The listing builds one solid part. Answer for the finished solid, in the listing's coordinates (mm). Round coordinates to 2 decimals unless told otherwise and drop trailing zeros. Write each loop counter-clockwise with the first axis right and the second up, starting at its lowest first coordinate (ties: lowest second). Pieces come first, ordered by that corner, then holes. Notation, with made-up numbers: (12.5, 37.5) - (49.5, 37.5) arc R17 cw to (49.5, 43.5) - close; hole circle Ø10 at (27.5, 58). An arc over 180 degrees is marked (long way). Return JSON: item names as keys, results as strings. Group by question number.
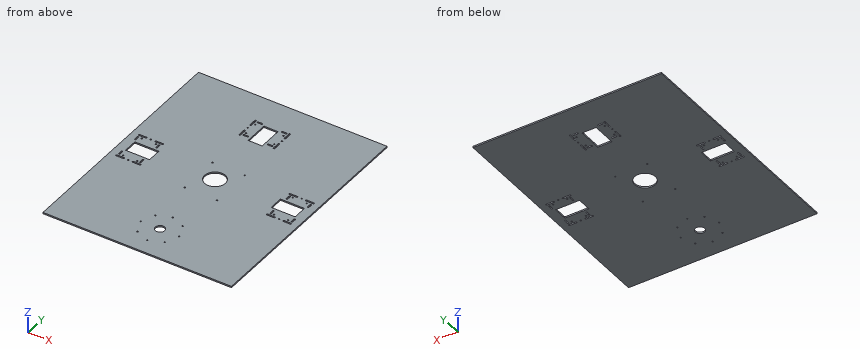
from build123d import *

# Parameters (mm, degrees)
SKETCH_1_W          = 400
SKETCH_1_H          = 500
SKETCH_1_R          = 1.5
SKETCH_1_R_2        = 22
SKETCH_1_R_3        = 10
SKETCH_1_W_2        = 30
SKETCH_1_H_2        = 51
SKETCH_1_W_3        = 51
SKETCH_1_H_3        = 30
EXTRUDE_1_DEPTH     = 3
SKETCH_2_R          = 1.5
CUT_EXTRUDE_1_DEPTH = 321.170267202


with BuildPart() as part:
    # 草图1 → 凸台-拉伸1 (new body)
    with BuildSketch(Plane.XY):
        Rectangle(SKETCH_1_W, SKETCH_1_H)
        with Locations((-36.4, 160)):
            Circle(SKETCH_1_R, mode=Mode.SUBTRACT)
        with Locations((-30, 145)):
            Circle(SKETCH_1_R, mode=Mode.SUBTRACT)
        with Locations((-30, 175)):
            Circle(SKETCH_1_R, mode=Mode.SUBTRACT)
        with Locations((36.4, 160)):
            Circle(SKETCH_1_R, mode=Mode.SUBTRACT)
        with Locations((30, 175)):
            Circle(SKETCH_1_R, mode=Mode.SUBTRACT)
        with Locations((30, 145)):
            Circle(SKETCH_1_R, mode=Mode.SUBTRACT)
        with Locations((160, -36.4)):
            Circle(SKETCH_1_R, mode=Mode.SUBTRACT)
        with Locations((145, -30)):
            Circle(SKETCH_1_R, mode=Mode.SUBTRACT)
        with Locations((175, -30)):
            Circle(SKETCH_1_R, mode=Mode.SUBTRACT)
        with Locations((160, 36.4)):
            Circle(SKETCH_1_R, mode=Mode.SUBTRACT)
        with Locations((175, 30)):
            Circle(SKETCH_1_R, mode=Mode.SUBTRACT)
        with Locations((145, 30)):
            Circle(SKETCH_1_R, mode=Mode.SUBTRACT)
        with Locations((-160, 36.4)):
            Circle(SKETCH_1_R, mode=Mode.SUBTRACT)
        with Locations((-145, 30)):
            Circle(SKETCH_1_R, mode=Mode.SUBTRACT)
        with Locations((-175, 30)):
            Circle(SKETCH_1_R, mode=Mode.SUBTRACT)
        with Locations((-160, -36.4)):
            Circle(SKETCH_1_R, mode=Mode.SUBTRACT)
        with Locations((-175, -30)):
            Circle(SKETCH_1_R, mode=Mode.SUBTRACT)
        with Locations((-145, -30)):
            Circle(SKETCH_1_R, mode=Mode.SUBTRACT)
        Circle(SKETCH_1_R_2, mode=Mode.SUBTRACT)
        with Locations((0, -176.690492226)):
            Circle(SKETCH_1_R_3, mode=Mode.SUBTRACT)
        with Locations((0, -135.985304682)):
            Circle(SKETCH_1_R, mode=Mode.SUBTRACT)
        with Locations((28.782914142, -147.907578084)):
            Circle(SKETCH_1_R, mode=Mode.SUBTRACT)
        with Locations((40.705187545, -176.690492226)):
            Circle(SKETCH_1_R, mode=Mode.SUBTRACT)
        with Locations((28.782914142, -205.473406369)):
            Circle(SKETCH_1_R, mode=Mode.SUBTRACT)
        with Locations((0, -217.395679771)):
            Circle(SKETCH_1_R, mode=Mode.SUBTRACT)
        with Locations((-28.782914142, -205.473406369)):
            Circle(SKETCH_1_R, mode=Mode.SUBTRACT)
        with Locations((-40.705187545, -176.690492226)):
            Circle(SKETCH_1_R, mode=Mode.SUBTRACT)
        with Locations((-28.782914142, -147.907578084)):
            Circle(SKETCH_1_R, mode=Mode.SUBTRACT)
        with BuildLine():
            Line((-34.8, 185), (-34.8, 170))
            ThreePointArc((-34.8, 170), (-36.4, 168.4), (-38, 170))
            Line((-38, 170), (-38, 185))
            ThreePointArc((-38, 185), (-36.4, 186.6), (-34.8, 185))
        make_face(mode=Mode.SUBTRACT)
        with BuildLine():
            Line((-38, 135), (-38, 150))
            ThreePointArc((-38, 150), (-36.4, 151.6), (-34.8, 150))
            Line((-34.8, 150), (-34.8, 135))
            ThreePointArc((-34.8, 135), (-36.4, 133.4), (-38, 135))
        make_face(mode=Mode.SUBTRACT)
        with BuildLine():
            Line((-22, 181.8), (-30, 181.8))
            ThreePointArc((-30, 181.8), (-31.6, 183.4), (-30, 185))
            Line((-30, 185), (-22, 185))
            ThreePointArc((-22, 185), (-20.4, 183.4), (-22, 181.8))
        make_face(mode=Mode.SUBTRACT)
        with BuildLine():
            Line((-30, 140), (-22, 140))
            ThreePointArc((-22, 140), (-20.4, 138.4), (-22, 136.8))
            Line((-22, 136.8), (-30, 136.8))
            ThreePointArc((-30, 136.8), (-31.6, 138.4), (-30, 140))
        make_face(mode=Mode.SUBTRACT)
        with BuildLine():
            Line((30, 140), (22, 140))
            ThreePointArc((22, 140), (20.4, 138.4), (22, 136.8))
            Line((22, 136.8), (30, 136.8))
            ThreePointArc((30, 136.8), (31.6, 138.4), (30, 140))
        make_face(mode=Mode.SUBTRACT)
        with BuildLine():
            Line((38, 135), (38, 150))
            ThreePointArc((38, 150), (36.4, 151.6), (34.8, 150))
            Line((34.8, 150), (34.8, 135))
            ThreePointArc((34.8, 135), (36.4, 133.4), (38, 135))
        make_face(mode=Mode.SUBTRACT)
        with BuildLine():
            Line((34.8, 185), (34.8, 170))
            ThreePointArc((34.8, 170), (36.4, 168.4), (38, 170))
            Line((38, 170), (38, 185))
            ThreePointArc((38, 185), (36.4, 186.6), (34.8, 185))
        make_face(mode=Mode.SUBTRACT)
        with BuildLine():
            Line((22, 181.8), (30, 181.8))
            ThreePointArc((30, 181.8), (31.6, 183.4), (30, 185))
            Line((30, 185), (22, 185))
            ThreePointArc((22, 185), (20.4, 183.4), (22, 181.8))
        make_face(mode=Mode.SUBTRACT)
        with Locations((0, 154.5)):
            Rectangle(SKETCH_1_W_2, SKETCH_1_H_2, mode=Mode.SUBTRACT)
        with Locations((154.5, 0)):
            Rectangle(SKETCH_1_W_3, SKETCH_1_H_3, mode=Mode.SUBTRACT)
        with BuildLine():
            Line((185, 34.8), (170, 34.8))
            ThreePointArc((170, 34.8), (168.4, 36.4), (170, 38))
            Line((170, 38), (185, 38))
            ThreePointArc((185, 38), (186.6, 36.4), (185, 34.8))
        make_face(mode=Mode.SUBTRACT)
        with BuildLine():
            Line((135, 38), (150, 38))
            ThreePointArc((150, 38), (151.6, 36.4), (150, 34.8))
            Line((150, 34.8), (135, 34.8))
            ThreePointArc((135, 34.8), (133.4, 36.4), (135, 38))
        make_face(mode=Mode.SUBTRACT)
        with BuildLine():
            Line((181.8, 22), (181.8, 30))
            ThreePointArc((181.8, 30), (183.4, 31.6), (185, 30))
            Line((185, 30), (185, 22))
            ThreePointArc((185, 22), (183.4, 20.4), (181.8, 22))
        make_face(mode=Mode.SUBTRACT)
        with BuildLine():
            Line((140, 30), (140, 22))
            ThreePointArc((140, 22), (138.4, 20.4), (136.8, 22))
            Line((136.8, 22), (136.8, 30))
            ThreePointArc((136.8, 30), (138.4, 31.6), (140, 30))
        make_face(mode=Mode.SUBTRACT)
        with BuildLine():
            Line((140, -30), (140, -22))
            ThreePointArc((140, -22), (138.4, -20.4), (136.8, -22))
            Line((136.8, -22), (136.8, -30))
            ThreePointArc((136.8, -30), (138.4, -31.6), (140, -30))
        make_face(mode=Mode.SUBTRACT)
        with BuildLine():
            Line((135, -38), (150, -38))
            ThreePointArc((150, -38), (151.6, -36.4), (150, -34.8))
            Line((150, -34.8), (135, -34.8))
            ThreePointArc((135, -34.8), (133.4, -36.4), (135, -38))
        make_face(mode=Mode.SUBTRACT)
        with BuildLine():
            Line((185, -34.8), (170, -34.8))
            ThreePointArc((170, -34.8), (168.4, -36.4), (170, -38))
            Line((170, -38), (185, -38))
            ThreePointArc((185, -38), (186.6, -36.4), (185, -34.8))
        make_face(mode=Mode.SUBTRACT)
        with BuildLine():
            Line((181.8, -22), (181.8, -30))
            ThreePointArc((181.8, -30), (183.4, -31.6), (185, -30))
            Line((185, -30), (185, -22))
            ThreePointArc((185, -22), (183.4, -20.4), (181.8, -22))
        make_face(mode=Mode.SUBTRACT)
        with Locations((-154.5, 0)):
            Rectangle(SKETCH_1_W_3, SKETCH_1_H_3, mode=Mode.SUBTRACT)
        with BuildLine():
            Line((-185, -34.8), (-170, -34.8))
            ThreePointArc((-170, -34.8), (-168.4, -36.4), (-170, -38))
            Line((-170, -38), (-185, -38))
            ThreePointArc((-185, -38), (-186.6, -36.4), (-185, -34.8))
        make_face(mode=Mode.SUBTRACT)
        with BuildLine():
            Line((-135, -38), (-150, -38))
            ThreePointArc((-150, -38), (-151.6, -36.4), (-150, -34.8))
            Line((-150, -34.8), (-135, -34.8))
            ThreePointArc((-135, -34.8), (-133.4, -36.4), (-135, -38))
        make_face(mode=Mode.SUBTRACT)
        with BuildLine():
            Line((-181.8, -22), (-181.8, -30))
            ThreePointArc((-181.8, -30), (-183.4, -31.6), (-185, -30))
            Line((-185, -30), (-185, -22))
            ThreePointArc((-185, -22), (-183.4, -20.4), (-181.8, -22))
        make_face(mode=Mode.SUBTRACT)
        with BuildLine():
            Line((-140, -30), (-140, -22))
            ThreePointArc((-140, -22), (-138.4, -20.4), (-136.8, -22))
            Line((-136.8, -22), (-136.8, -30))
            ThreePointArc((-136.8, -30), (-138.4, -31.6), (-140, -30))
        make_face(mode=Mode.SUBTRACT)
        with BuildLine():
            Line((-140, 30), (-140, 22))
            ThreePointArc((-140, 22), (-138.4, 20.4), (-136.8, 22))
            Line((-136.8, 22), (-136.8, 30))
            ThreePointArc((-136.8, 30), (-138.4, 31.6), (-140, 30))
        make_face(mode=Mode.SUBTRACT)
        with BuildLine():
            Line((-135, 38), (-150, 38))
            ThreePointArc((-150, 38), (-151.6, 36.4), (-150, 34.8))
            Line((-150, 34.8), (-135, 34.8))
            ThreePointArc((-135, 34.8), (-133.4, 36.4), (-135, 38))
        make_face(mode=Mode.SUBTRACT)
        with BuildLine():
            Line((-185, 34.8), (-170, 34.8))
            ThreePointArc((-170, 34.8), (-168.4, 36.4), (-170, 38))
            Line((-170, 38), (-185, 38))
            ThreePointArc((-185, 38), (-186.6, 36.4), (-185, 34.8))
        make_face(mode=Mode.SUBTRACT)
        with BuildLine():
            Line((-181.8, 22), (-181.8, 30))
            ThreePointArc((-181.8, 30), (-183.4, 31.6), (-185, 30))
            Line((-185, 30), (-185, 22))
            ThreePointArc((-185, 22), (-183.4, 20.4), (-181.8, 22))
        make_face(mode=Mode.SUBTRACT)
    extrude(amount=EXTRUDE_1_DEPTH)

    # 草图2 → 切除-拉伸1 (cut, through all)
    with BuildSketch(Plane.XY.offset(3)):
        with Locations((-31, 39.03)):
            Circle(SKETCH_2_R)
        with Locations((37.45, 39.03)):
            Circle(SKETCH_2_R)
        with Locations((-31, -50)):
            Circle(SKETCH_2_R)
        with Locations((37.45, -50)):
            Circle(SKETCH_2_R)
    extrude(amount=-CUT_EXTRUDE_1_DEPTH, mode=Mode.SUBTRACT)


solid = part.part
(1) A flat-ended cylindrical pin translates along its axis: pin 1 (1.8 mm diameter, centred on x = 28.78, y = -147.91, fed in from -Z). Find the tip coordinate at first contact, or state that the pin passes through.
(2) Consider line 1 (Y direction, x = -36.4, z = 1); line 2 (X direction, y = 147, z = 1.4); line 3 (Y direction, x = 0, z = 0.75). Determine where each line is inside the solid, lowest interval first.
(3) Find section B-B (z = 2.1). State how many separate pieces and enclosed holes the cut face has, plus the area to 3 significant figures.
(4) Find section A-A (y = 0). Write down the section's boundary in (x, z), plus the area to 3 significant figures.
Check sheet entries:
{
 "1": {"pin 1": "passes through"},
 "2": {"line 1": "y = -250 to 133.4, 151.6 to 158.5, 161.5 to 168.4, 186.6 to 250", "line 2": "x = -200 to -38, -34.8 to -15, 15 to 34.8, 38 to 200", "line 3": "y = -250 to -218.9, -215.9 to -186.69, -166.69 to -137.49, -134.49 to -22, 22 to 129, 180 to 250"},
 "3": {"separate pieces": "1", "enclosed holes": "59", "area": "192,000 mm^2"},
 "4": {"outline": "(-200, 0) - (-180, 0) - (-180, 3) - (-200, 3) - close; (-129, 0) - (-22, 0) - (-22, 3) - (-129, 3) - close; (22, 0) - (129, 0) - (129, 3) - (22, 3) - close; (180, 0) - (200, 0) - (200, 3) - (180, 3) - close", "area": "762 mm^2"}
}
